Work out the finished part from the listing and answer in its coordinate system (mm). A direction names the side the tool comes from. Coordinates: 2 decimals unless noted, no trailing zeros. Order: outer loops, then holes, each group sorted by start corner. A loop starts at its lowest first (then second) coordinate and runs counter-clockwise, first axis right, second up.
1. The part is cut by section A-A, the plane x = 0. Give the vertices of the cut face in (y, z), then the cut area to 3 significant figures.
2. Determine the mould class of faces 4 (the flat face through (-5, 7.62, 5)), 5 (the cylindrical face through (11.333, 9.498, -1.488)), 6 (the cylindrical face through (0.596, 5.531, 2.685)) for opening direction X: +X half, -X half, draft (parallel to the pull), parting line (faces both ways), or undercut.
3. The part is cut by section D-D, the plane y = 10.5. Give the vertices of the cut face in (x, z).
4. The part is cut by section B-B, the plane z = 0. Give the vertices of the cut face in (x, y), then the cut area to 3 significant figures.
5. The part is cut by section C-C, the plane y = 3.5. Give the vertices of the cut face in (x, z).
6. Flat-ended cylindrical pins translate along their axes: pin 1 Ø4 at (x, y) = (-6, 3) entering from -Z; pin 2 Ø2 at (x, y) = (-4, 4.5) entering from -Z; pin 3 Ø4.5 at (x, z) = (0, 0) entering from +Y; pin 4 Ø4 at (x, y) = (3, 5.5) entering from -Z. Find the tip coordinate at first contact, or state that the pin passes through.
7. Find the intervals of material crossed by probe 1 along Z at (x, y) = (0, 3.5); probe 2 along Y at (x, z) = (-4.5, 6.5); probe 3 along X at (y, z) = (6.75, -1), in increasing order.
8. A tool of negligible diameter and unlimited length cuts with its end or side. For faces 1 (the cylindrical face through (-3.86, 3.76, -5.04)), 2 (the flat face through (2.3, 11.22, 2.3)), 3 (the flat face through (-4, 13.97, 4)), from which of +Z, -Z, +X, -X, +Y, -Y can it reach the whole face along a straight path? Write none if from no direction.
```python
from build123d import *

# Parameters (mm, degrees)
SKETCH1_R                       = 6.35
BOSS_EXTRUDE1_DEPTH             = 8.89
BOSS_EXTRUDE2_DEPTH             = 5.08
BOSS_EXTRUDE2_DEPTH_BACK        = 1.27
SKETCH2_R                       = 11.43
CBORE_FOR_M5_SBHCS1_D           = 5.5
CBORE_FOR_M5_SBHCS1_CBORE_D     = 10.5
CBORE_FOR_M5_SBHCS1_CBORE_DEPTH = 2.75
FILLET1_R                       = 2.54


with BuildPart() as part:
    # Sketch1 → Boss-Extrude1 (new body)
    with BuildSketch(Plane(origin=(0, 0, 0), x_dir=(1, 0, 0), z_dir=(0, 1, 0))):
        with Locations(Location((0, 0, 0), (0, 0, 270))):
            Circle(SKETCH1_R)
    extrude(amount=BOSS_EXTRUDE1_DEPTH)

    # Sketch2 → Boss-Extrude2 (add, two sides: drawn at the far end of the back side and taken through both)
    with BuildSketch(Plane(origin=(0, 8.89, 0), x_dir=(1, 0, 0), z_dir=(0, 1, 0)).offset(-BOSS_EXTRUDE2_DEPTH_BACK)):
        with Locations(Location((0, 0, 0), (0, 0, 270))):
            Circle(SKETCH2_R)
    extrude(amount=BOSS_EXTRUDE2_DEPTH + BOSS_EXTRUDE2_DEPTH_BACK)

    # CBORE for M5 SBHCS1 (through all)
    with Locations(Plane(origin=(0, 13.97, 0), x_dir=(1, 0, 0), z_dir=(0, 1, 0))):
        with Locations((0, 0)):
            CounterBoreHole(CBORE_FOR_M5_SBHCS1_D / 2, CBORE_FOR_M5_SBHCS1_CBORE_D / 2, CBORE_FOR_M5_SBHCS1_CBORE_DEPTH)

    # Fillet1
    fillet1_edges = [part.edges().sort_by_distance(p)[0] for p in [
        (0, 13.97, -11.43),
    ]]
    fillet(fillet1_edges, radius=FILLET1_R)


solid = part.part
```
Geometry says:
1. outline: (0, -6.35) - (7.62, -6.35) - (7.62, -11.43) - (11.43, -11.43) arc R2.54 ccw to (13.97, -8.89) - (13.97, -5.25) - (11.22, -5.25) - (11.22, -2.75) - (0, -2.75) - close; (0, 2.75) - (11.22, 2.75) - (11.22, 5.25) - (13.97, 5.25) - (13.97, 8.89) arc R2.54 ccw to (11.43, 11.43) - (7.62, 11.43) - (7.62, 6.35) - (0, 6.35) - close
1. area: 149 mm2
2. face 4: draft
2. face 5: parting line
2. face 6: undercut
3. outline: circle Ø22.86 at (0, 0); hole circle Ø5.5 at (0, 0)
4. outline: (-11.43, 7.62) - (-6.35, 7.62) - (-6.35, 0) - (-2.75, 0) - (-2.75, 11.22) - (-5.25, 11.22) - (-5.25, 13.97) - (-8.89, 13.97) arc R2.54 ccw to (-11.43, 11.43) - close; (2.75, 0) - (6.35, 0) - (6.35, 7.62) - (11.43, 7.62) - (11.43, 11.43) arc R2.54 ccw to (8.89, 13.97) - (5.25, 13.97) - (5.25, 11.22) - (2.75, 11.22) - close
4. area: 149 mm2
5. outline: circle Ø12.7 at (0, 0); hole circle Ø5.5 at (0, 0)
6. pin 1: stops at z = -4.93
6. pin 2: stops at z = -5.6
6. pin 3: passes through
6. pin 4: stops at z = -6.27
7. probe 1: z = -6.35 to -2.75, 2.75 to 6.35
7. probe 2: y = 7.62 to 13.97
7. probe 3: x = -6.27 to -2.56, 2.56 to 6.27
8. face 1: -Y
8. face 2: +Y
8. face 3: +Z, -Z, +X, -X, +Y
